```python
from build123d import *

# Parameters (mm, degrees)
F1_DEPTH = 1.524


with BuildPart() as f1:
    # F0 (on Top) → F1 (new body)
    with BuildSketch(Plane.XY):
        Polygon((-97.248423, -135.78557), (-66.097785, -162.864407), (145.052415, -162.864407), (166.070805, -134.972061), align=None)
        Polygon((-330.176573, 66.695782), (-97.248423, -135.78557), (166.070805, -134.972061), (319.55103, 68.703076), align=None)
        Polygon((-362.728536, 94.992772), (-330.176573, 66.695782), (319.55103, 68.703076), (339.361736, 94.992772), align=None)
    extrude(amount=F1_DEPTH)


solid = f1.part
```
Source: CAD feature listing. Evaluate the final solid. Frame: model axes, mm. Coordinates: 2 decimals unless noted, no trailing zeros. Loops run counter-clockwise (first coordinate to the right, second up) from the corner with the lowest first, then second, coordinate; pieces in that order, holes last. Notation, with made-up numbers: M -35.75,49.5 L -25.75,49.5 A23 ccw -25.75,88.5 Z; hole C -28,-37.5 d5. An arc over 180 degrees is marked long. Put each result on its own line as item: value. Start each with the question number.
1) Cut plane B-B on x = 190.5. Return the cut outline in (y, z).
2) Cut plane C-C on y = -109.5. Return the cut outline in (x, z).
3) Cut plane A-A on z = 0.45. Return the cut outline in (x, y).
4) Ray query, L1, parallel to X at y = -22.5, z = 1.1; L2, parallel to Y at x = -81.5, z = 0.2; L3, parallel to Y at x = 297, z = 0.8. Return the intervals inside material, ascending. Write a range as from..to.
The answers:
1. outline: M -102.55,0 L 94.99,0 L 94.99,1.52 L -102.55,1.52 Z
2. outline: M -127.49,0 L 185.27,0 L 185.27,1.52 L -127.49,1.52 Z
3. outline: M -362.73,94.99 L -66.1,-162.86 L 145.05,-162.86 L 339.36,94.99 Z
4. L1: x = -227.57..250.82
4. L2: y = -149.48..94.99
4. L3: y = 38.78..94.99
